Autodesk Inventor part; units mm, degrees
ref_plane "YZ Plane" through (0, 0, 0) normal (1, 0, 0) x (0, 1, 0)
ref_plane "XZ Plane" through (0, 0, 0) normal (0, 1, 0) x (-1, 0, 0)
ref_plane "XY Plane" through (0, 0, 0) normal (0, 0, 1) x (1, 0, 0)
sketch "스케치1" plane through (0, 0, 0) normal (0, 0, 1) x (1, 0, 0)
  line L0 (26.8403, -18.2471) -> (-26.8403, -18.2471)
  line L1 (-26.8403, -18.2471) -> (-26.8403, 18.2471)
  line L2 (-26.8403, 18.2471) -> (26.8403, 18.2471)
  line L3 (26.8403, 18.2471) -> (26.8403, -18.2471)
  line L4 (26.8403, -18.2471) -> (-26.8403, 18.2471) construction
  line L5 (-26.8403, -18.2471) -> (26.8403, 18.2471) construction
  point P0 (0, 0)
extrude "돌출1" add sketch "스케치1" along normal blind 50
sketch "스케치2" plane through (-26.8403, 18.2471, 0) normal (0, 1, 0) x (1, 0, 0)
  line L0 (0, -50) -> (53.6805, -50)
  line L1 (0, -50) -> (20, -50)
  line L2 (20, -50) -> (20, -34)
  line L3 (20, -34) -> (0, -34)
  line L4 (0, -34) -> (0, -50)
  line L5 (0, 0) -> (20, 0)
  line L6 (20, 0) -> (20, -16)
  line L7 (20, -16) -> (0, -16)
  line L8 (0, -16) -> (0, 0)
  line L9 (20, -34) -> (38, -34)
  line L10 (38, -34) -> (38, -16)
  line L11 (38, -16) -> (20, -16)
  line L12 (20, -16) -> (20, -34)
  line L13 (38, -34) -> (53.6805, -34)
  line L14 (53.6805, -34) -> (53.6805, -50)
  line L15 (53.6805, -50) -> (38, -50)
  line L16 (38, -50) -> (38, -34)
  line L17 (53.6805, 0) -> (53.6805, -50)
  line L18 (38, -16) -> (53.6805, -16)
  line L19 (53.6805, -16) -> (53.6805, 0)
  line L20 (53.6805, 0) -> (38, 0)
  line L21 (38, 0) -> (38, -16)
  point P0 (26.8403, 0)
  dimension "d2" = 20
  dimension "d3" = 16
  dimension "d4" = 20
  dimension "d5" = 16
  dimension "d6" = 18
extrude "돌출2" cut sketch "스케치2" against normal blind 10 contours L4 L3 L2 L0 | L7 L8 L5 L6
extrude "돌출3" cut sketch "스케치2" against normal blind 15 contours L12 L11 L10 L9
extrude "돌출4" cut sketch "스케치2" against normal blind 50 contours L16 L13 L14 L0 | L21 L20 L17 L18
sketch "스케치3" plane through (11.1597, 18.2471, 34) normal (0, 0, 1) x (1, 0, 0)
  line L0 (15.6805, -36.4941) -> (15.6805, 0)
  line L1 (0, -15) -> (15.6805, -36.4941)
  line L2 (15.6805, -36.4941) -> (15.6805, 0)
  line L3 (0, -36.4941) -> (0, 0)
  line L4 (15.6805, 0) -> (0, 0)
  line L5 (0, 0) -> (0, -15)
  point P0 (-11.1597, -18.2471)
extrude "돌출5" cut sketch "스케치3" against normal blind 50
sketch "스케치4" plane through (0, 0, 50) normal (0, 0, 1) x (1, 0, 0)
  line L0 (-6.8403, 8.2471) -> (-6.8403, 18.2471)
  line L1 (-6.8403, 3.2471) -> (11.1597, 3.2471)
  line L2 (-6.8403, 8.2471) -> (11.1597, 3.2471)
  line L3 (11.1597, 18.2471) -> (-6.8403, 18.2471)
  line L4 (11.1597, 3.2471) -> (11.1597, 18.2471)
  line L5 (11.1597, 18.2471) -> (-6.8403, 18.2471)
  line L6 (-6.8403, 18.2471) -> (-6.8403, 8.2471)
  point P0 (0, 0)
extrude "돌출6" cut sketch "스케치4" against normal blind 50
sketch "스케치5" plane through (0, 0, 50) normal (0, 0, 1) x (1, 0, 0)
  line L0 (-26.8403, 8.2471) -> (-26.8403, -18.2471)
  line L1 (-26.8403, -18.2471) -> (11.1597, -18.2471)
  line L2 (-26.8403, -10.3165) -> (-15.6784, -10.3165)
  line L3 (-15.6784, -10.3165) -> (-15.6784, -18.2471)
  line L4 (-15.6784, -18.2471) -> (-26.8403, -18.2471)
  line L5 (-26.8403, -18.2471) -> (-26.8403, -10.3165)
  point P0 (0, 0)
extrude "돌출7" cut sketch "스케치5" against normal blind 50
properties part number "240628_final1"
Could you check a few things on this model? Use its own coordinates, in mm. A direction names the side the tool comes from. Give positions to 0.01 mm unless a question says otherwise; leave off trailing zeros. Order: outer loops, then holes, each group sorted by start corner. A loop starts at its lowest first (then second) coordinate and runs counter-clockwise, first axis right, second up.
Q1. Suppose I cut it at B-B, the plane x = -14. Write out the boundary of the cut face in (y, z), and give its area (3 significant figures).
Q2. If I drill on line 1 along Z through (x, y) = (-12.5, 10.5); line 2 along X through (y, z) = (-1, 4.5); line 3 along Y through (x, z) = (10, 20), over which ranges is the centre line in solid material (lowest first)?
Q3. We'd pull the mould along Z, two halves only. Please class faces 6 (the flat face through (17, -10, 16)), 7 (the flat face through (-17, 18.247, 25)), 8 (the flat face through (-2, 5, 16)), 9 (the flat face through (15, -12, 34)): +Z half, -Z half, draft (parallel to the pull), parting line (faces both ways), or undercut.
Q4. Suppose I cut it at A-A, the plane z = 39. Write out the boundary of the cut face in (x, y).
Q5. I'm going to push flat-ended pins straight in: P1, Ø1, axis at x = -7.5, y = 9.5, coming from the +Z side; P2, Ø4, axis at y = -15.5, z = 24, coming from the -X side; P3, Ø4, axis at x = -0.5, y = 4.5, coming from the -Z side; P4, Ø5, axis at y = -12.5, z = 45, coming from the +X side. Where does each tip first touch, or does it pass through?
Q6. For faces 1 (the flat face through (2, 3.247, 25)), 2 (the flat face through (-15.678, -14, 25)), 3 (the flat face through (-17, 13, 16)), 4 (the flat face through (-17, 13, 34)), 5 (the flat face through (11.16, -7, 8)), which set-ups out of +Z, -Z, +X, -X, +Y, -Y let a thin tool reach every point of the face, with its end or its side?
Q7. Suppose I cut it at D-D, the plane y = 11.5. Write out the boundary of the cut face in (x, z), and give its area (3 significant figures).
Q8. Suppose I cut it at C-C, the plane y = -12. Write out the boundary of the cut face in (x, z), and give its area (3 significant figures).
Solution:
1. outline: (-18.25, 0) - (8.25, 0) - (8.25, 16) - (18.25, 16) - (18.25, 34) - (8.25, 34) - (8.25, 50) - (-18.25, 50) - close
1. area: 1,500 mm2
2. line 1: z = 16 to 34
2. line 2: x = -26.84 to 11.16
2. line 3: y = -18.25 to 3.25
3. face 6: -Z half
3. face 7: draft
3. face 8: undercut
3. face 9: +Z half
4. outline: (-26.84, -10.32) - (-15.68, -10.32) - (-15.68, -18.25) - (11.16, -18.25) - (11.16, 3.25) - (-6.84, 8.25) - (-26.84, 8.25) - close
5. P1: stops at z = 34
5. P2: stops at x = -15.68
5. P3: stops at z = 0
5. P4: stops at x = 11.16
6. face 1: +X, +Y
6. face 2: +Z, -Z, -X, -Y
6. face 3: -Z, +X, -X, +Y
6. face 4: +Z, +X, -X, +Y
6. face 5: -Z, +X, +Y, -Y
7. outline: (-26.84, 16) - (-6.84, 16) - (-6.84, 34) - (-26.84, 34) - close
7. area: 360 mm2
8. outline: (-15.68, 0) - (11.16, 0) - (11.16, 16) - (22.28, 16) - (22.28, 34) - (11.16, 34) - (11.16, 50) - (-15.68, 50) - close
8. area: 1,540 mm2
